Geometry check sheet. Reference: the model listing, model coordinates, mm. A direction names the side the tool comes from. Give positions to 0.01 mm unless a question says otherwise; leave off trailing zeros. Write each loop counter-clockwise with the first axis right and the second up, starting at its lowest first coordinate (ties: lowest second). Pieces come first, ordered by that corner, then holes. Notation, with made-up numbers: (-6, 60.25) -> (45, 60.25) arc R35 ccw to (45, 97.25) -> close; hole circle Ø1 at (-0.5, -7.75). An arc over 180 degrees is marked (long way). One line per item, written item: value.
from build123d import *

# Parameters (mm, degrees)
SKETCH1_W           = 90
SKETCH1_H           = 100
BOSS_EXTRUDE1_DEPTH = 3
SKETCH2_R           = 1.7
CUT_EXTRUDE1_DEPTH  = 4
SKETCH4_W           = 81.2
SKETCH4_H           = 93.2
SKETCH4_W_2         = 75.2
SKETCH4_H_2         = 87.2
BOSS_EXTRUDE2_DEPTH = 2
CUT_EXTRUDE5_START  = -3
SKETCH6_R           = 6
CUT_EXTRUDE5_DEPTH  = 3
SKETCH7_W           = 90
SKETCH7_H           = 3
BOSS_EXTRUDE3_DEPTH = 4
SKETCH8_R           = 3.75
BOSS_EXTRUDE4_DEPTH = 3
FILLET1_R           = 8


with BuildPart() as part:
    # Sketch1 → Boss-Extrude1 (new body)
    with BuildSketch(Plane(origin=(0, 0, 0), x_dir=(1, 0, 0), z_dir=(0, 1, 0))):
        Rectangle(SKETCH1_W, SKETCH1_H)
    extrude(amount=BOSS_EXTRUDE1_DEPTH)

    # Sketch2 → Cut-Extrude1 (cut, through all)
    with BuildSketch(Plane(origin=(0, 3, 0), x_dir=(1, 0, 0), z_dir=(0, 1, 0))):
        with Locations((-39, 44)):
            Circle(SKETCH2_R)
        with Locations((39, 44)):
            Circle(SKETCH2_R)
        with Locations((39, -44)):
            Circle(SKETCH2_R)
        with Locations((-39, -44)):
            Circle(SKETCH2_R)
    extrude(amount=-CUT_EXTRUDE1_DEPTH, mode=Mode.SUBTRACT)

    # Sketch4 → Boss-Extrude2 (add)
    with BuildSketch(Plane.XZ):
        with Locations((1, 0)):
            Rectangle(SKETCH4_W, SKETCH4_H)
        with Locations((1, 0)):
            Rectangle(SKETCH4_W_2, SKETCH4_H_2, mode=Mode.SUBTRACT)
    extrude(amount=BOSS_EXTRUDE2_DEPTH)

    # Sketch6 → Cut-Extrude5 (cut, through all)
    with BuildSketch(Plane(origin=(0, 3, 0), x_dir=(1, 0, 0), z_dir=(0, 1, 0)).offset(CUT_EXTRUDE5_START)):
        with Locations((-39, 44)):
            Circle(SKETCH6_R)
        with Locations((-39, -44)):
            Circle(SKETCH6_R)
        with Locations((39, -44)):
            Circle(SKETCH6_R)
        with Locations((39, 44)):
            Circle(SKETCH6_R)
    extrude(amount=-CUT_EXTRUDE5_DEPTH, mode=Mode.SUBTRACT)

    # Sketch7 → Boss-Extrude3 (add)
    with BuildSketch(Plane.XY.offset(50)):
        with Locations((0, 1.5)):
            Rectangle(SKETCH7_W, SKETCH7_H)
    extrude(amount=BOSS_EXTRUDE3_DEPTH)

    # Sketch8 → Boss-Extrude4 (add)
    with BuildSketch(Plane(origin=(0, 3, 0), x_dir=(1, 0, 0), z_dir=(0, 1, 0))):
        Polygon((-45, -50), (-45, -54), (45, -54), (45, -50), (45, 50), (-45, 50), align=None)
        with Locations((-39, 44)):
            Circle(SKETCH8_R, mode=Mode.SUBTRACT)
        with Locations((39, 44)):
            Circle(SKETCH8_R, mode=Mode.SUBTRACT)
        with Locations((-39, -44)):
            Circle(SKETCH8_R, mode=Mode.SUBTRACT)
        with Locations((39, -44)):
            Circle(SKETCH8_R, mode=Mode.SUBTRACT)
    extrude(amount=BOSS_EXTRUDE4_DEPTH)

    # Fillet1
    fillet1_edges = [part.edges().sort_by_distance(p)[0] for p in [
        (-45, 3, 54),
        (45, 3, 54),
        (-45, 3, -50),
        (45, 3, -50),
    ]]
    fillet(fillet1_edges, radius=FILLET1_R)


solid = part.part
1) Tool access check on faces 4 (the flat face through (-1, 3, 54)), 5 (the cylindrical face through (36.024, 4.479, 46.282)). Record the directions out of +Z, -Z, +X, -X, +Y, -Y that give a thin tool (end or side, any length) a straight path to the whole face; none if there is none.
Verdict:
face 4: +Z, +X, -X, +Y, -Y
face 5: +Y
2) Sectioned sample at A-A on x = 25.5. Record the cut outline in (y, z).
Verdict:
outline: (-2, -46.6) -> (0, -46.6) -> (0, -50) -> (6, -50) -> (6, 54) -> (0, 54) -> (0, 46.6) -> (-2, 46.6) -> (-2, 43.6) -> (0, 43.6) -> (0, -43.6) -> (-2, -43.6) -> close
3) Sectioned sample at B-B on z = -25.5. Record the cut outline in (x, y).
Verdict:
outline: (-45, 0) -> (-39.6, 0) -> (-39.6, -2) -> (-36.6, -2) -> (-36.6, 0) -> (38.6, 0) -> (38.6, -2) -> (41.6, -2) -> (41.6, 0) -> (45, 0) -> (45, 6) -> (-45, 6) -> close
4) Mould release check, pull along Z, two halves, no side actions. Record for faces 1 (the cylindrical face through (-42.594, 2.958, -47.719)), 2 (the cylindrical face through (42.594, 3.042, 51.719)), 3 (the cylindrical face through (-39.81, 4.48, -40.34)): released by +Z, released by -Z, zero draft, split by the parting line, or undercut.
Verdict:
face 1: released by -Z
face 2: released by +Z
face 3: undercut
5) Scan lines: probe 1 along X at (y, z) = (4.7, 44); probe 2 along Z at (x, y) = (-39, 0.75); probe 3 along Z at (x, y) = (39, 4). Record each from-to range of solid material in increasing order.
Verdict:
probe 1: -45 to -42.75, -35.25 to 35.25, 42.75 to 45
probe 2: -49.75 to -45.7, -42.3 to 42.3, 45.7 to 53.75
probe 3: -49.75 to -47.75, -40.25 to 40.25, 47.75 to 53.75
6) Depth check by flat-ended pin: pin 1 Ø4.5 at (x, z) = (-39, -44) entering from -Y; pin 2 Ø1.6 at (x, y) = (-10, -1.5) entering from -Z; pin 3 Ø4.5 at (x, z) = (39, 44) entering from +Y. Enter the tip coordinate at first touch or a pass-through.
Verdict:
pin 1: y = 0
pin 2: z = -46.6
pin 3: y = 3
